Work out the finished part from the listing and answer in its coordinate system (mm). A direction names the side the tool comes from. Round coordinates to 2 decimals unless told otherwise and drop trailing zeros. Order: outer loops, then holes, each group sorted by start corner. A loop starts at its lowest first (then second) coordinate and runs counter-clockwise, first axis right, second up. Notation, with made-up numbers: M -37,-7 L -16,-7 A21 cw -16,13 Z; hole C 67,85.25 d1. An arc over 180 degrees is marked long. Return JSON: item names as keys, results as strings.
from build123d import *

# Parameters (mm, degrees)
BOSS_EXTRUDE1_DEPTH    = 300
CAP_SCREW1_D           = 3.5
CAP_SCREW1_CBORE_D     = 6
CAP_SCREW1_CBORE_DEPTH = 4.5
SCALE_2_SCALE          = 1.7


with BuildPart() as part:
    # Sketch1 → Boss-Extrude1 (new body)
    with BuildSketch(Plane(origin=(-20, 0, 0), x_dir=(0, 0, -1), z_dir=(1, 0, 0))):
        with BuildLine():
            Line((6.5, 12.5), (7.5, 11.5))
            Line((7.5, 11.5), (7.5, 10))
            ThreePointArc((7.5, 10), (7.220600207, 9.128142709), (6.486486486, 8.581081081))
            ThreePointArc((6.486486486, 8.581081081), (5.059724666, 5.990862007), (7.5, 4.320550528))
            Line((7.5, 4.320550528), (7.5, 0.5))
            Line((7.5, 0.5), (7, 0))
            Line((7, 0), (-7, 0))
            Line((-7, 0), (-7.5, 0.5))
            Line((-7.5, 0.5), (-7.5, 4.320550528))
            ThreePointArc((-7.5, 4.320550528), (-5.059724666, 5.990862007), (-6.486486486, 8.581081081))
            ThreePointArc((-6.486486486, 8.581081081), (-7.220600207, 9.128142709), (-7.5, 10))
            Line((-7.5, 10), (-7.5, 11.5))
            Line((-7.5, 11.5), (-6.5, 12.5))
            Line((-6.5, 12.5), (6.5, 12.5))
        make_face()
    extrude(amount=BOSS_EXTRUDE1_DEPTH)

    # Cap Screw1 (through all)
    with Locations(Plane(origin=(0, 12.5, 0), x_dir=(1, 0, 0), z_dir=(0, 1, 0))):
        with Locations((0, 0), (60, 0), (120, 0), (180, 0), (240, 0), (300, 0), (360, 0), (420, 0)):
            CounterBoreHole(CAP_SCREW1_D / 2, CAP_SCREW1_CBORE_D / 2, CAP_SCREW1_CBORE_DEPTH)


with BuildPart() as part_1:
    # 缩放比例2: scaled about (0, 0, 0)
    add(part.part.scale(SCALE_2_SCALE))


solid = part_1.part
Item 1: Consider line 1 along Y through (x, z) = (151.5, 9.5); line 2 along Z through (x, y) = (306, 6) (3 decimals); line 3 along Z through (x, y) = (306, 10.5) (3 decimals). Determine where each line is inside the solid, lowest interval first. Write a range as [from, to].
Output:
{"line 1": "y = [0, 8.5], [13.6, 21.25]", "line 2": "z = [-12.75, -2.975], [2.975, 12.75]", "line 3": "z = [-8.541, -2.975], [2.975, 8.541]"}
Item 2: Find section A-A (x = 278). Determine the outline of the cut face in (y, z).
Output:
{"outline": "M 0,-11.9 L 0.85,-12.75 L 7.34,-12.75 A3.74 cw 14.59,-11.03 A2.55 ccw 17,-12.75 L 19.55,-12.75 L 21.25,-11.05 L 21.25,11.05 L 19.55,12.75 L 17,12.75 A2.55 ccw 14.59,11.03 A3.74 cw 7.34,12.75 L 0.85,12.75 L 0,11.9 Z"}
Item 3: The mould has two halves that part along Z. Classify faces 1 (the flat face through (3.3, 13.6, -0.1)), 2 (the flat face through (217, 0, 0)): pulls with the +Z half, pulls with the -Z half, needs draft (parallel to the pull), parting line crosses it, or undercut.
Output:
{"face 1": "undercut", "face 2": "needs draft"}
Item 4: Which of the six approach directions +Z, -Z, +X, -X, +Y, -Y give full straight-line access (tool end or side, diameter ignored) to faces 3 (the flat face through (476, 11, 0)), 4 (the flat face through (101.9, 13.6, 3.3))?
Output:
{"face 3": "+Z, -Z, +X, +Y, -Y", "face 4": "+Y"}
Item 5: Each of these flat-tipped pins is pushed along its axis until it touches: pin 1 (1.5 mm diameter, centred on x = 129.5, z = 2, fed in from -Y); pin 2 (8 mm diameter, centred on x = 204, z = 0, fed in from +Y); pin 3 (1.5 mm diameter, centred on x = 121, y = 10, fed in from +Z); pin 4 (5 mm diameter, centred on x = 381, y = 14, fed in from +Z). Where does it stop, or does it pass through?
Output:
{"pin 1": "stops at y = 0", "pin 2": "stops at y = 13.6", "pin 3": "stops at z = 8.96", "pin 4": "stops at z = 12.7"}
